Can you work these out from the model? Positions are in its coordinate system, mm. A direction names the side the tool comes from. Give positions to 0.01 mm unless a question says otherwise; leave off trailing zeros. Loops run counter-clockwise (first coordinate to the right, second up) from the corner with the lowest first, then second, coordinate; pieces in that order, holes last. Notation, with made-up numbers: (74.25, 67.5) - (122.25, 67.5) arc R8 cw to (122.25, 74.5) - close; hole circle Ø1 at (66, -4). An arc over 180 degrees is marked (long way). Answer as a JSON object with one key per item and string values. Group by question number.
Item 1: Suppose I cut it at B-B on y = 106.5. Write out the boundary of the cut face in (x, z), and give its area (3 significant figures).
Item 2: Suppose I cut it at A-A on x = 8. Write out the boundary of the cut face in (y, z).
Item 3: Which directions (+Z, -Z, +X, -X, +Y, -Y) give clear straight access to the entire face, cutting with the end or side of a thin tool? Please do faces 1 (the flat face through (0, -11, -8.66)), 2 (the flat face through (-2.768, 49.3, 1.556)), 3 (the flat face through (0, 111, -8.66)).
Item 4: Thinking about a two-plate mould opening in Y: for faces 4 (the flat face through (2.73, 49.3, 1.62)), 5 (the flat face through (0, 111, 7.585)), 6 (the flat face through (0, 0, 4)), 7 (the cylindrical face through (0, -19, 8)), which applies, pulls with the +Y half, pulls with the -Y half, needs draft (parallel to the pull), parting line crosses it, or undercut?
Item 5: Please list where these lines run through material, in increasing order: L1, parallel to Y at x = 0, z = 8.45; L2, parallel to Z at x = 2.25, y = -5; L3, parallel to Y at x = 0.25, z = -5.
Item 6: Will these pins go through, and if not, where does the flat tip stop? pin 1 (12 mm diameter, centred on y = 55.5, z = 2.5, fed in from +X); pin 2 (2 mm diameter, centred on x = -5, z = -7.5, fed in from +Y); pin 3 (0.9 mm diameter, centred on y = -7.5, z = -8, fed in from -X).
from build123d import *

# Parameters (mm, degrees)
BOSS_EXTRUDE1_DEPTH = 100
SKETCH3_R           = 10
BOSS_EXTRUDE2_DEPTH = 4
SKETCH5_W           = 10
SKETCH5_H           = 1.075357982
BOSS_EXTRUDE3_DEPTH = 15
FILLET3_RADIUS      = 5
FILLET3_LENGTH      = 1.075357982
FILLET4_RADIUS      = 5
FILLET4_LENGTH      = 1.075357982
CUT_EXTRUDE1_REACH  = 122.869
SKETCH6_R           = 1


with BuildPart() as part:
    # Sketch2 → Boss-Extrude1 (new body)
    with BuildSketch(Plane(origin=(0, 0, 0), x_dir=(1, 0, 0), z_dir=(0, 1, 0))):
        Polygon((1.843695467, 3.168851584), (-1.822458239, 3.181112903), (-3.666153706, 0.012261319), (-1.843695467, -3.168851584), (1.822458239, -3.181112903), (3.666153706, -0.012261319), align=None)
    extrude(amount=BOSS_EXTRUDE1_DEPTH)

    # Sketch3 → Boss-Extrude2 (add)
    with BuildSketch(Plane(origin=(0, 100, 0), x_dir=(1, 0, 0), z_dir=(0, 1, 0))):
        with Locations(Location((0, 0, 0), (0, 0, 270))):
            Circle(SKETCH3_R)
    extrude(amount=BOSS_EXTRUDE2_DEPTH)

    # Sketch5 → Boss-Extrude3 (add)
    with BuildSketch(Plane(origin=(0, 104, 0), x_dir=(1, 0, 0), z_dir=(0, 1, 0))):
        with Locations((0, 8.122575047)):
            Rectangle(SKETCH5_W, SKETCH5_H)
        with Locations((0, -8.122575047)):
            Rectangle(SKETCH5_W, SKETCH5_H)
    extrude(amount=BOSS_EXTRUDE3_DEPTH)

    # Fillet3: full round fillet: the end face becomes a half cylinder, R = half its width
    fillet3_face = Plane((0, 119, 8.122575047), x_dir=(0, 0, -1), z_dir=(0, 1, 0))  # on the end face: x along it, z out of the body
    fillet3_slab = fillet3_face.offset(-FILLET3_RADIUS / 2) * Box(FILLET3_LENGTH, 2 * FILLET3_RADIUS, FILLET3_RADIUS, mode=Mode.PRIVATE)  # the body's end, R deep
    fillet3_round = Plane((0, 114, 8.122575047), x_dir=(0, 1, 0), z_dir=(0, 0, -1)) * Cylinder(FILLET3_RADIUS, FILLET3_LENGTH, mode=Mode.PRIVATE)  # its axis R under the face
    add(fillet3_slab - fillet3_round, mode=Mode.SUBTRACT)

    # Fillet4: full round fillet: the end face becomes a half cylinder, R = half its width
    fillet4_face = Plane((0, 119, -8.122575047), x_dir=(0, 0, 1), z_dir=(0, 1, 0))  # on the end face: x along it, z out of the body
    fillet4_slab = fillet4_face.offset(-FILLET4_RADIUS / 2) * Box(FILLET4_LENGTH, 2 * FILLET4_RADIUS, FILLET4_RADIUS, mode=Mode.PRIVATE)  # the body's end, R deep
    fillet4_round = Plane((0, 114, -8.122575047), x_dir=(0, 1, 0), z_dir=(0, 0, 1)) * Cylinder(FILLET4_RADIUS, FILLET4_LENGTH, mode=Mode.PRIVATE)  # its axis R under the face
    add(fillet4_slab - fillet4_round, mode=Mode.SUBTRACT)

    # Cut-Extrude1: up to this face of the body (flat: up to its plane)
    cut_extrude1_end = Plane(part.part.faces().sort_by_distance((0, 111.008207501, -8.660254038))[0])
    # Sketch6 → Cut-Extrude1 (cut, up to the picked face)
    with BuildSketch(Plane.XY.offset(8.660254038), mode=Mode.PRIVATE) as cut_extrude1_sk1:
        with Locations((0, 114)):
            Circle(SKETCH6_R)
    cut_extrude1_tool1 = split(extrude(cut_extrude1_sk1.sketch, amount=-CUT_EXTRUDE1_REACH, mode=Mode.PRIVATE), bisect_by=cut_extrude1_end, keep=Keep.BOTH, mode=Mode.PRIVATE)
    add(cut_extrude1_tool1.solids().sort_by(Axis((0, 114, 8.660254), (0, 0, -1)))[0], mode=Mode.SUBTRACT)

    # Mirror1: part across plane


with BuildPart() as part_1:
    add(part.part)
    add(part.part.mirror(Plane(origin=(0, 50, 0), x_dir=(0, 0, 1), z_dir=(0, -1, 0))))


solid = part_1.part
Worked out:
{
 "1": {"outline": "(-5, -8.66) - (5, -8.66) - (5, -7.58) - (-5, -7.58) - close; (-5, 7.58) - (5, 7.58) - (5, 8.66) - (-5, 8.66) - close", "area": "21.5 mm2"},
 "2": {"outline": "(-4, -6) - (0, -6) - (0, 6) - (-4, 6) - close; (100, -6) - (104, -6) - (104, 6) - (100, 6) - close"},
 "3": {"face 1": "-Z, +X, -X, -Y", "face 2": "+Z, -X", "face 3": "-Z, +X, -X, +Y"},
 "4": {"face 4": "undercut", "face 5": "needs draft", "face 6": "undercut", "face 7": "pulls with the -Y half"},
 "5": {"L1": "y = -19 to -15, -13 to 0, 100 to 113, 115 to 119", "L2": "z = -8.66 to -7.58, 7.58 to 8.66", "L3": "y = -4 to 0, 100 to 104"},
 "6": {"pin 1": "stops at x = 3.67", "pin 2": "stops at y = 117", "pin 3": "stops at x = -5"}
}
